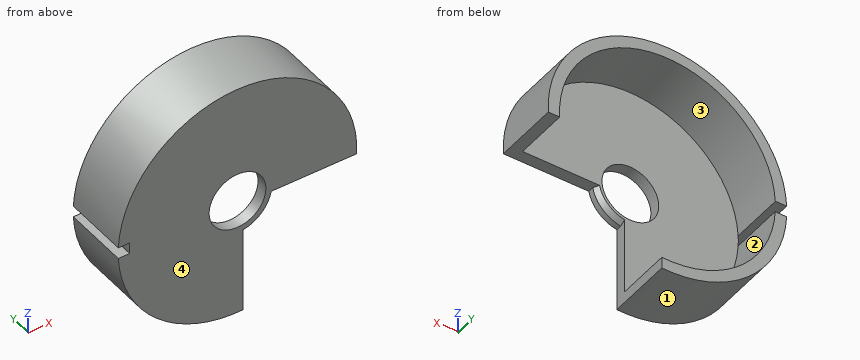
Autodesk Inventor part; units mm, degrees
ref_plane "YZ Plane" through (0, 0, 0) normal (1, 0, 0) x (0, 1, 0)
ref_plane "XZ Plane" through (0, 0, 0) normal (0, 1, 0) x (-1, 0, 0)
ref_plane "XY Plane" through (0, 0, 0) normal (0, 0, 1) x (1, 0, 0)
sketch "Sketch9" plane through (0, 0, 0) normal (0, 1, 0) x (-1, 0, 0)
  line L0 (21, 0) -> (-21, 0) construction
  line L1 (0, 21) -> (0, -21) construction
  line L2 (21, -1) -> (20.9762, -1)
  line L3 (21, 1) -> (20.9762, 1)
  line L4 (-20.9762, 1) -> (-21, 1)
  line L5 (1, 21) -> (1, 20.9762)
  line L6 (1, -20.9762) -> (1, -21)
  line L7 (-1, 21) -> (-1, 20.9762)
  line L8 (-1, -5.9161) -> (-1, -21)
  line L9 (-5.9161, -1) -> (-18.9762, -1)
  circle A0 centre (0, 0) radius 5
  arc A1 (-5.9161, -1) -> (-1, -5.9161) centre (0, 0) ccw
  line L10 (-20.9762, -1) -> (-18.9762, -1)
  line L11 (1, -21) -> (1, -3.873) construction
  line L12 (-3.873, 1) -> (-18.9762, 1) construction
  line L13 (-18.9762, 1) -> (-20.9762, 1) construction
  line L14 (-3.873, 1) -> (20.9762, 1) construction
  line L15 (-5.9161, -1) -> (20.9762, -1) construction
  line L16 (1, -3.873) -> (1, 20.9762) construction
  line L17 (-1, -5.9161) -> (-1, 20.9762) construction
  line L18 (0, 21) -> (0, 19) construction
  line L19 (0, 19) -> (1, 19) construction
  arc A2 (-1, -20.9762) -> (0, 21) centre (0, 0) ccw construction
  arc A3 (20.9762, 1) -> (-20.9762, -1) centre (0, 0) ccw construction
  arc A4 (-1, -18.9737) -> (-18.9737, -1) centre (0, 0) ccw
  line L20 (-1, 19) -> (1, 19)
  point P0 (-4.899, -1)
  point P1 (-1, -4.899)
  dimension "d35" = 10
  dimension "d50" = 2
  dimension "d53" = 38
extrude "Extrusion5" add sketch "Sketch9" along normal blind 2
chamfer "Chamfer1" distance 0.5 distance2 1 1 edges at (4.2426, 2, -4.2426) measured on face at (13.5988, 2, 4.219)
sketch "Sketch12" plane through (0, 0, 0) normal (0, 1, 0) x (-1, 0, 0)
  circle A0 centre (0, 0) radius 5
  arc A1 (-1, -18.9737) -> (-18.9737, -1) centre (0, 0) ccw
  line L0 (-18.9737, -1) -> (-5.4083, -1)
  line L1 (-18.9737, -1) -> (-20.9762, -1)
  line L2 (-1, -5.4083) -> (-1, -18.9737)
  line L3 (-1, -18.9737) -> (-1, -20.9762)
  line L4 (-20.9762, -1) -> (20.9762, -1) construction
  line L5 (-20.9762, 1) -> (20.9762, 1) construction
  line L6 (20.9762, 1) -> (18.9762, 1)
  line L7 (20.9762, -1) -> (18.9762, -1)
  line L8 (18.9762, -1) -> (18.9762, 1)
  arc A2 (-1, -20.9762) -> (20.9762, -1) centre (0, 0) ccw
  arc A3 (20.9762, 1) -> (-20.9762, -1) centre (0, 0) ccw
  point P0 (18.9762, 0.9512)
  point P1 (18.9762, -0.9512)
  dimension "d60" = 19
  dimension "d63" = 2
  dimension "d64" = 2
  dimension "d65" = 2
extrude "Extrusion8" add sketch "Sketch12" along normal blind 11.5 contours A1 L1 A3 L6 L8 | A1 L8 L7 A2 L3
properties part number "base layer 3"
Model file for the job. Use its own axes, mm. Face numbers are marked on the shaded views. Round coordinates to 2 decimals unless told otherwise and drop trailing zeros. Loops run counter-clockwise (first coordinate to the right, second up) from the corner with the lowest first, then second, coordinate; pieces in that order, holes last. Notation, with made-up numbers: (75.25, 44) - (112.25, 44) arc R28 ccw to (112.25, 83) - close; hole circle Ø3 at (-35.75, 25). An arc over 180 degrees is marked (long way). Write each question's results on one line, items separated by ' | '.
(1) Wall check: L1, parallel to Z at x = 0, y = 1.3; L2, parallel to Y at x = -4, z = 13.5; L3, parallel to X at y = 8.5, z = 14. Give the ranges that are in metal, low to high.
Answer below:
L1: z = -21 to -5, 5 to 21 | L2: y = 0 to 2 | L3: x = -15.65 to -12.85, 12.85 to 15.65
(2) Saw through at B-B, the plane z = 0. List the corners of the cut face in (x, y).
Answer below:
outline: (-19, 0) - (-5, 0) - (-5, 2) - (-19, 2) - close; (5, 0) - (21, 0) - (21, 11.5) - (19, 11.5) - (19, 2) - (5, 2) - close
(3) Pin check, flat tips, straight feed: pin 1 (2 mm diameter, centred on x = -20, y = 7.5, fed in from -Z); pin 2 (3.5 mm diameter, centred on y = 4, z = -12.5, fed in from +X); pin 3 (1.6 mm diameter, centred on x = -20, y = 5.5, fed in from +Z); pin 4 (1 mm diameter, centred on x = 2, z = -12.5, fed in from +Y). Stop position of each tip, or through.
Answer below:
pin 1: stops at z = -8.94 | pin 2: stops at x = -12.57 | pin 3: stops at z = 8.51 | pin 4: passes through
(4) Saw through at A-A, the plane x = 0. List the corners of the cut face in (y, z), then the cut area to 3 significant figures.
Answer below:
outline: (0, -21) - (11.5, -21) - (11.5, -19) - (2, -19) - (2, -5) - (0, -5) - close; (0, 5) - (2, 5) - (2, 19) - (11.5, 19) - (11.5, 21) - (0, 21) - close | area: 102 mm^2
(5) Saw through at C-C, the plane y = 6.5. List the corners of the cut face in (x, z).
Answer below:
outline: (-20.98, -1) arc R21 ccw to (1, -20.98) - (1, -18.97) arc R19 cw to (-18.98, -0.95) - (-18.98, -1) - close; (-20.98, 1) - (-18.98, 1) - (-18.98, 0.95) arc R19 cw to (18.97, -1) - (20.98, -1) arc R21 ccw to start
(6) Mould opens along Z. For the marked faces 1, 2, 3 and 4 say: released by +Z, released by -Z, zero draft, split by the parting line, or undercut.
Answer below:
face 1: released by -Z | face 2: undercut | face 3: undercut | face 4: zero draft
(7) Saw through at D-D, the plane z = 15.5. List the corners of the cut face in (x, y), then the cut area to 3 significant figures.
Answer below:
outline: (-14.17, 0) - (14.17, 0) - (14.17, 11.5) - (10.99, 11.5) - (10.99, 2) - (-10.99, 2) - (-10.99, 11.5) - (-14.17, 11.5) - close | area: 117 mm^2
